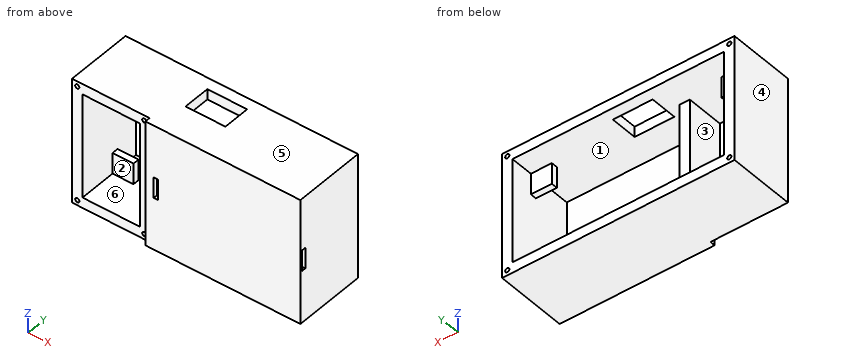
```python
from build123d import *

# Parameters (mm, degrees)
SKETCH1_W           = 111
SKETCH1_H           = 60
BOSS_EXTRUDE1_DEPTH = 34.5
SKETCH2_W           = 101
SKETCH2_H           = 50
CUT_EXTRUDE1_DEPTH  = 11
CUT_EXTRUDE3_DEPTH  = 14
CUT_EXTRUDE5_START  = -2
SKETCH5_W           = 27.5
SKETCH5_H           = 50
SKETCH5_W_2         = 68.5
CUT_EXTRUDE5_DEPTH  = 18.5
SKETCH6_W           = 37
SKETCH6_H           = 60
CUT_EXTRUDE6_DEPTH  = 2.5
SKETCH7_R           = 1
CUT_EXTRUDE7_DEPTH  = 4
SKETCH8_R           = 1
CUT_EXTRUDE8_DEPTH  = 4
SKETCH9_W           = 19
SKETCH9_H           = 13
CUT_EXTRUDE9_DEPTH  = 10
SKETCH10_W          = 10
SKETCH10_H          = 2
CUT_EXTRUDE10_DEPTH = 70
SKETCH11_W          = 2
SKETCH11_H          = 10
CUT_EXTRUDE11_DEPTH = 2


with BuildPart() as part:
    # Sketch1 → Boss-Extrude1 (new body)
    with BuildSketch(Plane(origin=(0, 0, 0), x_dir=(1, 0, 0), z_dir=(0, 1, 0))):
        with Locations((55.5, 30)):
            Rectangle(SKETCH1_W, SKETCH1_H)
    extrude(amount=BOSS_EXTRUDE1_DEPTH)

    # Sketch2 → Cut-Extrude1 (cut)
    with BuildSketch(Plane(origin=(0, 34.5, 0), x_dir=(1, 0, 0), z_dir=(0, 1, 0))):
        with Locations((55.5, 30)):
            Rectangle(SKETCH2_W, SKETCH2_H)
    extrude(amount=-CUT_EXTRUDE1_DEPTH, mode=Mode.SUBTRACT)

    # Sketch3 → Cut-Extrude3 (cut)
    with BuildSketch(Plane(origin=(0, 34.5, 0), x_dir=(1, 0, 0), z_dir=(0, 1, 0))):
        Polygon((5, 45), (15, 45), (15, 55), (96, 55), (96, 45), (106, 45), (106, 15), (96, 15), (96, 5), (15, 5), (15, 15), (5, 15), align=None)
    extrude(amount=-CUT_EXTRUDE3_DEPTH, mode=Mode.SUBTRACT)

    # Sketch5 → Cut-Extrude5 (cut)
    with BuildSketch(Plane.XZ.offset(CUT_EXTRUDE5_START)):
        with Locations((18.75, -30)):
            Rectangle(SKETCH5_W, SKETCH5_H)
        with Locations((71.75, -30)):
            Rectangle(SKETCH5_W_2, SKETCH5_H)
    extrude(amount=-CUT_EXTRUDE5_DEPTH, mode=Mode.SUBTRACT)

    # Sketch6 → Cut-Extrude6 (cut)
    with BuildSketch(Plane.XZ):
        with Locations((18.5, -30)):
            Rectangle(SKETCH6_W, SKETCH6_H)
    extrude(amount=-CUT_EXTRUDE6_DEPTH, mode=Mode.SUBTRACT)

    # Sketch7 → Cut-Extrude7 (cut)
    with BuildSketch(Plane(origin=(0, 2.5, 0), x_dir=(-1, 0, 0), z_dir=(0, -1, 0))):
        with Locations((-2.5, 57.5)):
            Circle(SKETCH7_R)
        with Locations((-34.5, 57.5)):
            Circle(SKETCH7_R)
        with Locations((-34.5, 2.5)):
            Circle(SKETCH7_R)
        with Locations((-2.5, 2.5)):
            Circle(SKETCH7_R)
    extrude(amount=-CUT_EXTRUDE7_DEPTH, mode=Mode.SUBTRACT)

    # Sketch8 → Cut-Extrude8 (cut)
    with BuildSketch(Plane(origin=(0, 34.5, 0), x_dir=(1, 0, 0), z_dir=(0, 1, 0))):
        with Locations((2.5, 57.5)):
            Circle(SKETCH8_R)
        with Locations((108.5, 57.5)):
            Circle(SKETCH8_R)
        with Locations((108.5, 2.360383006)):
            Circle(SKETCH8_R)
        with Locations((2.5, 2.5)):
            Circle(SKETCH8_R)
    extrude(amount=-CUT_EXTRUDE8_DEPTH, mode=Mode.SUBTRACT)

    # Sketch9 → Cut-Extrude9 (cut)
    with BuildSketch(Plane.XY):
        with Locations((52.792502494, 22.713514363)):
            Rectangle(SKETCH9_W, SKETCH9_H)
    extrude(amount=-CUT_EXTRUDE9_DEPTH, mode=Mode.SUBTRACT)

    # Sketch10 → Cut-Extrude10 (cut)
    with BuildSketch(Plane(origin=(111, 0, 0), x_dir=(0, 0, -1), z_dir=(1, 0, 0))):
        with Locations((30, 2)):
            Rectangle(SKETCH10_W, SKETCH10_H)
    extrude(amount=-CUT_EXTRUDE10_DEPTH, mode=Mode.SUBTRACT)

    # Sketch11 → Cut-Extrude11 (cut, through all)
    with BuildSketch(Plane(origin=(0, 1, 0), x_dir=(1, 0, 0), z_dir=(0, 1, 0))):
        with Locations((42, 30)):
            Rectangle(SKETCH11_W, SKETCH11_H)
    extrude(amount=-CUT_EXTRUDE11_DEPTH, mode=Mode.SUBTRACT)


solid = part.part
```
For this review, take the finished solid that the model builds, in its own axes (mm). Face numbers are marked on the shaded views. A direction names the side the tool comes from. Round coordinates to 2 decimals unless told otherwise and drop trailing zeros. Write each loop counter-clockwise with the first axis right and the second up, starting at its lowest first coordinate (ties: lowest second). Pieces come first, ordered by that corner, then holes. Notation, with made-up numbers: (53, 82) -> (88, 82) arc R30 ccw to (88, 104) -> close; hole circle Ø2 at (-40, 43). An arc over 180 degrees is marked (long way). One line per question, with ' | ' between items. Start each with the question number.
(1) Tool access review of the marked faces 1, 2 and 3: name each direction out of +Z, -Z, +X, -X, +Y, -Y from which nothing blocks a thin tool from reaching the whole face with its end or side.
(2) Add section D-D, the plane z = -29. Write out the cut boundary in (x, y), plus the area to 3 significant figures.
(3) Mouldability with a two-part tool opening along X and no side actions: class the marked faces 4, 5 and 6 as released by +X, released by -X, zero draft, split by the parting line, or undercut.
(4) Add section A-A, the plane x = 13. Write out the cut boundary in (y, z), plus the area to 3 significant figures.
(5) For line 1 along Z through (x, y) = (2.5, 4.45); line 2 along X through (y, z) = (4, -27.5); line 3 along X through (y, z) = (5.6, -2.5), list the stretches that pass through material, from the lowest coordinate up. Write a range as from..to.
(6) Add section C-C, the plane y = 14. Write out the cut boundary in (x, z).
(7) Insertion check: P1, Ø1.8, axis at x = 2.5, z = -2.5, coming from the +Y side; P2, Ø3, axis at x = 103, z = -50.5, coming from the +Y side; P3, Ø3, axis at x = 9.5, z = -52.5, coming from the -Y side. Each pin has a flat end and moves straight along its axis. Give the tip position at first contact, or say it passes through.
(8) Add section B-B, the plane z = -49.5. Write out the cut boundary in (x, y).
Answer list:
1) face 1: none | face 2: -Y | face 3: +Y, -Y
2) outline: (0, 2.5) -> (5, 2.5) -> (5, 34.5) -> (0, 34.5) -> close; (32.5, 2.5) -> (37, 2.5) -> (37, 0) -> (41, 0) -> (41, 2) -> (37.5, 2) -> (37.5, 20.5) -> (32.5, 20.5) -> close; (43, 0) -> (111, 0) -> (111, 1) -> (43, 1) -> close; (106, 3) -> (111, 3) -> (111, 34.5) -> (106, 34.5) -> close | area: 484 mm²
3) face 4: released by -X | face 5: zero draft | face 6: undercut
4) outline: (2.5, -60) -> (34.5, -60) -> (34.5, -55) -> (23.5, -55) -> (23.5, -45) -> (20.5, -45) -> (20.5, -55) -> (2.5, -55) -> close; (2.5, -5) -> (20.5, -5) -> (20.5, -15) -> (23.5, -15) -> (23.5, -5) -> (34.5, -5) -> (34.5, 0) -> (2.5, 0) -> close | area: 380 mm²
5) line 1: -60..-58.5, -56.5..-3.5, -1.5..0 | line 2: 0..5, 32.5..37.5, 106..111 | line 3: 0..1.5, 3.5..33.5, 35.5..111
6) outline: (0, -60) -> (111, -60) -> (111, 0) -> (0, 0) -> close; hole (5, -55) -> (32.5, -55) -> (32.5, -5) -> (5, -5) -> close; hole (37.5, -55) -> (106, -55) -> (106, -5) -> (37.5, -5) -> close
7) P1: y = 30.5 | P2: y = 23.5 | P3: y = 20.5
8) outline: (0, 2.5) -> (5, 2.5) -> (5, 20.5) -> (15, 20.5) -> (15, 23.5) -> (5, 23.5) -> (5, 34.5) -> (0, 34.5) -> close; (32.5, 2.5) -> (37, 2.5) -> (37, 0) -> (111, 0) -> (111, 34.5) -> (106, 34.5) -> (106, 23.5) -> (96, 23.5) -> (96, 20.5) -> (106, 20.5) -> (106, 2) -> (37.5, 2) -> (37.5, 20.5) -> (32.5, 20.5) -> close
